The listing builds one solid part. Answer for the finished solid, in the listing's coordinates (mm). A direction names the side the tool comes from. Give positions to 0.01 mm unless a question says otherwise; leave off trailing zeros. Loops run counter-clockwise (first coordinate to the right, second up) from the corner with the lowest first, then second, coordinate; pieces in that order, holes last. Notation, with made-up numbers: (28, -30) - (36, -30) arc R24 cw to (36, -12) - close; hole circle Ø7 at (86.5, 38.25). An arc over 180 degrees is marked (long way). Write item = value, one per line. Start each with the question number.
1) Which of the six approach directions +Z, -Z, +X, -X, +Y, -Y give full straight-line access (tool end or side, diameter ignored) to faces 4 (the cylindrical face through (-7.25, 8.43, -98.75)), 5 (the cylindrical face through (-67.76, -0.64, -133.56)), 6 (the cylindrical face through (78.72, -20.54, -118.94)), 7 (the cylindrical face through (15.494, -1.143, -145.047))?
2) Consider probe 1 along X at (y, z) = (5.5, -130.5); probe 2 along Z at (x, y) = (103, -1); probe 3 along X at (y, z) = (-12, -141). Determine where each line is inside the solid, lowest interval first.
3) The part is cut by section A-A on x = -29. Write down the section's boundary in (y, z), plus the area to 3 significant figures.
4) The mould has two halves that part along X. Classify faces 1 (the cylindrical face through (-38.408, 6.703, -102.907)), 2 (the flat face through (-66.279, 15, -119)), 3 (the flat face through (-104.279, 0, -119)): +X half, -X half, draft (parallel to the pull), parting line (faces both ways), or undercut.
5) Flat-ended cylindrical pins translate along their axes: P1, Ø3.5, axis at x = 56, y = -20, coming from the +Z side; P2, Ø3, axis at y = -0.5, z = -101, coming from the -X side; P3, Ø2, axis at x = 59, y = -19.5, coming from the -Z side. Find the tip coordinate at first contact, or state that the pin passes through.
from build123d import *

# Parameters (mm, degrees)
SKETCH_1_W          = 15
SKETCH_1_H          = 12
SKETCH_1_W_2        = 3
SKETCH_1_H_2        = 10.5
SKETCH_1_H_3        = 14.5
SKETCH_1_H_4        = 17
SKETCH_1_H_5        = 22.5
CHAMFER_1_SIZE      = 1
CUT_EXTRUDE_1_DEPTH = 4
CUT_EXTRUDE_2_DEPTH = 5
SKETCH_5_W          = 16
SKETCH_5_H          = 6
CUT_EXTRUDE_3_DEPTH = 3


with BuildPart() as part:
    # 草图1 → 旋转1 (revolve)
    with BuildSketch(Plane(origin=(0, 0, 0), x_dir=(1, 0, 0), z_dir=(0, 1, 0))):
        with Locations((-96.778500263, 113.072139402)):
            Rectangle(SKETCH_1_W, SKETCH_1_H)
        with Locations((-87.778500263, 113.822139402)):
            Rectangle(SKETCH_1_W_2, SKETCH_1_H_2)
        Polygon((-69.278500263, 119.072139402), (-69.278500263, 104.072139402), (-86.278500263, 104.072139402), (-86.278500263, 108.572139402), (-86.278500263, 119.072139402), align=None)
        with Locations((-67.778500263, 111.822139402)):
            Rectangle(SKETCH_1_W_2, SKETCH_1_H_3)
        Polygon((-66.278500263, 119.072139402), (-66.278500263, 104.572139402), (-66.278500263, 101.572139402), (-12.278500263, 101.572139402), (-12.278500263, 102.072139402), (-12.278500263, 119.072139402), align=None)
        with Locations((-10.778500263, 110.572139402)):
            Rectangle(SKETCH_1_W_2, SKETCH_1_H_4)
        Polygon((-5.278500263, 119.072139402), (-9.278500263, 119.072139402), (-9.278500263, 102.072139402), (-9.278500263, 97.072139402), (-5.278500263, 97.072139402), align=None)
        Polygon((34.721499737, 119.072139402), (-5.278500263, 119.072139402), (-5.278500263, 97.072139402), (-5.278500263, 93.072139402), (34.721499737, 93.072139402), (34.721499737, 96.572139402), align=None)
        with Locations((36.221499737, 107.822139402)):
            Rectangle(SKETCH_1_W_2, SKETCH_1_H_5)
        Polygon((87.721499737, 119.072139402), (37.721499737, 119.072139402), (37.721499737, 96.572139402), (37.721499737, 96.072139402), (87.721499737, 96.072139402), (87.721499737, 102.072139402), align=None)
        with Locations((89.221499737, 110.572139402)):
            Rectangle(SKETCH_1_W_2, SKETCH_1_H_4)
        Polygon((138.721499737, 119.072139402), (90.721499737, 119.072139402), (90.721499737, 102.072139402), (90.721499737, 101.572139402), (138.721499737, 101.572139402), (138.721499737, 104.257707549), (138.721499737, 107.072139402), (138.721499737, 108.572139402), align=None)
        with Locations((140.221499737, 113.822139402)):
            Rectangle(SKETCH_1_W_2, SKETCH_1_H_2)
        Polygon((154.721499737, 119.072139402), (141.721499737, 119.072139402), (141.721499737, 108.572139402), (141.721499737, 107.072139402), (154.721499737, 107.072139402), align=None)
    revolve(axis=Axis((-109.712030386, 0, -119.072139402), (1, 0, 0)))

    # 倒角1
    chamfer_1_edges = [part.edges().sort_by_distance(p)[0] for p in [
        (-104.278500263, 0, -131.072139402),
        (154.721499737, 0, -131.072139402),
        (138.721499737, 0, -136.572139402),
        (87.721499737, 0, -142.072139402),
        (-5.278500263, 0, -145.072139402),
        (-66.278500263, 0, -136.572139402),
        (-86.278500263, 0, -134.072139402),
    ]]
    chamfer(chamfer_1_edges, length=CHAMFER_1_SIZE)

    # 草图2 → 切除-拉伸1 (cut)
    with BuildSketch(Plane(origin=(0, -15, 0), x_dir=(-1, 0, 0), z_dir=(0, -1, 0))):
        with BuildLine():
            Line((78.278500263, 115.072139402), (76.278500263, 115.072139402))
            ThreePointArc((76.278500263, 115.072139402), (72.278500263, 119.072139402), (76.278500263, 123.072139402))
            Line((76.278500263, 123.072139402), (78.278500263, 123.072139402))
            ThreePointArc((78.278500263, 123.072139402), (82.278500263, 119.072139402), (78.278500263, 115.072139402))
        make_face()
    extrude(amount=-CUT_EXTRUDE_1_DEPTH, mode=Mode.SUBTRACT)

    # 草图3 → 切除-拉伸2 (cut)
    with BuildSketch(Plane(origin=(0, -23, 0), x_dir=(-1, 0, 0), z_dir=(0, -1, 0))):
        with BuildLine():
            Line((-48.721499737, 113.072139402), (-72.721499737, 113.072139402))
            ThreePointArc((-72.721499737, 113.072139402), (-78.721499737, 119.072139402), (-72.721499737, 125.072139402))
            Line((-72.721499737, 125.072139402), (-48.721499737, 125.072139402))
            ThreePointArc((-48.721499737, 125.072139402), (-42.721499737, 119.072139402), (-48.721499737, 113.072139402))
        make_face()
    extrude(amount=-CUT_EXTRUDE_2_DEPTH, mode=Mode.SUBTRACT)

    # 草图5 → 切除-拉伸3 (cut)
    with BuildSketch(Plane(origin=(0, -12, 0), x_dir=(-1, 0, 0), z_dir=(0, -1, 0))):
        with Locations((-146.728951344, 119.072139402)):
            Rectangle(SKETCH_5_W, SKETCH_5_H)
    extrude(amount=-CUT_EXTRUDE_3_DEPTH, mode=Mode.SUBTRACT)


solid = part.part
Answer below:
q1.face_4 = -X
q1.face_5 = none
q1.face_6 = -Y
q1.face_7 = +X, -X
q2.probe_1 = -86.28 to 138.72
q2.probe_2 = -136.54 to -101.6
q2.probe_3 = -5.28 to 34.72
q3.outline = circle Ø35 at (0, -119.07)
q3.area = 962 mm2
q4.face_1 = draft
q4.face_2 = undercut
q4.face_3 = -X half
q5.P1 = -105.07
q5.P2 = -66.2
q5.P3 = -132.74
